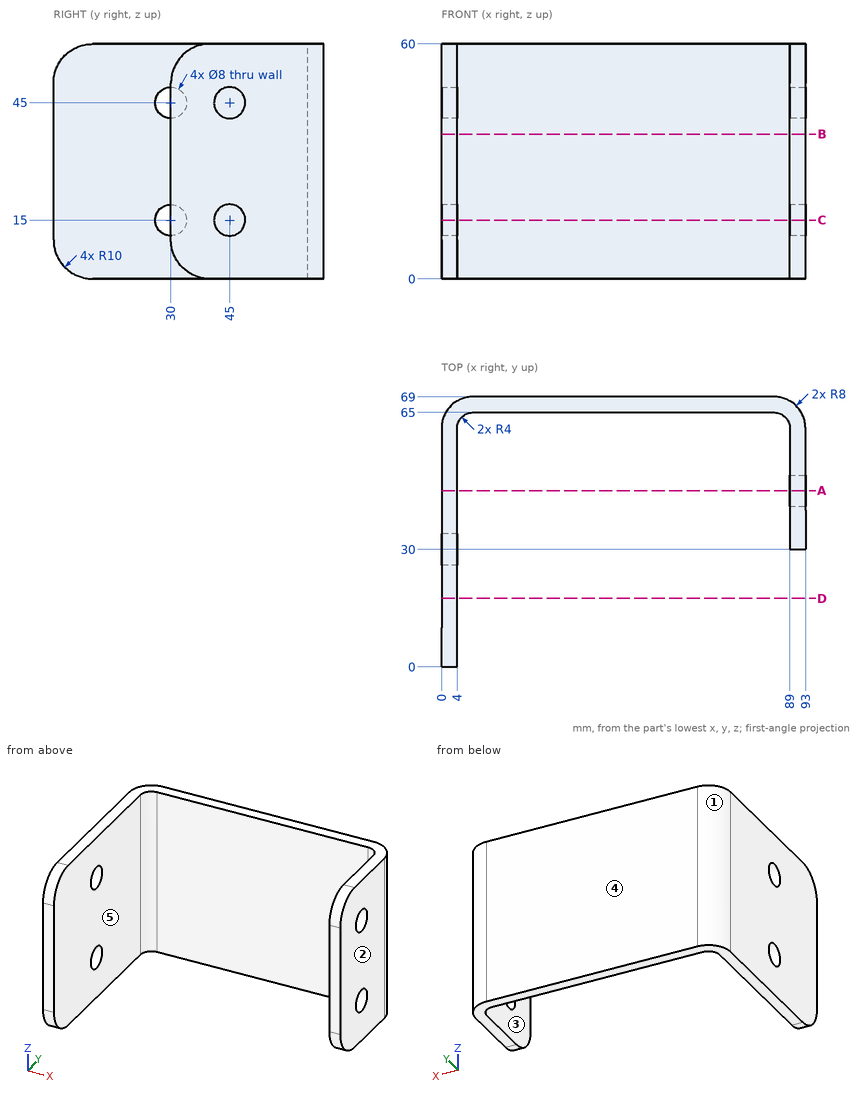
Geometry check sheet. Reference: drawing and pictorial views, mm from the part's lowest x, y, z. A direction names the side the tool comes from. Give positions to 0.01 mm unless a question says otherwise; leave off trailing zeros. Write each loop counter-clockwise with the first axis right and the second up, starting at its lowest first coordinate (ties: lowest second). Pieces come first, ordered by that corner, then holes.
Item 1: Cross-section at B-B (z = 37). Enter the section's corners in (x, y).
Item 2: Gauge pin test, flat ends, axial feed: pin 1 (6 mm diameter, centred on x = 40.5, z = 53.5, fed in from -Y); pin 2 (6.5 mm diameter, centred on y = 30, z = 45, fed in from -X); pin 3 (1 mm diameter, centred on y = 24.5, z = 40, fed in from +X). Record the tip position at first contact, or that the pin passes through.
Item 3: Access from +Z, -Z, +X, -X, +Y, -Y to the whole of each face (thin tool, end or side, straight path). Record for the marked faces 4 and 5.
Item 4: Cross-section at D-D (y = 17.5). Enter the section's corners in (x, z), and give its area (3 significant figures).
Item 5: Cross-section at C-C (z = 15). Enter the section's corners in (x, y).
Item 6: Draft check along X on the marked faces 1, 2 and 3. Enter one of: released by +X, released by -X, zero draft, split by the parting line, or undercut.
Item 7: Scan lines: L1, parallel to X at y = 45, z = 4.5; L2, parallel to X at y = 28.5, z = 29.5; L3, parallel to Y at x = 91, z = 45. Record each from-to range of solid material in increasing order.
Item 8: Cross-section at A-A (y = 45). Enter the section's corners in (x, z), and give its area (3 significant figures).
Report:
1. outline: (0, 0) - (4, 0) - (4, 61) arc R4 cw to (8, 65) - (85, 65) arc R4 cw to (89, 61) - (89, 30) - (93, 30) - (93, 61) arc R8 ccw to (85, 69) - (8, 69) arc R8 ccw to (0, 61) - close
2. pin 1: stops at y = 65
2. pin 2: stops at x = 89
2. pin 3: stops at x = 4
3. face 4: +Z, -Z, +X, -X, +Y
3. face 5: +Z, -Z, -Y
4. outline: (0, 0) - (4, 0) - (4, 60) - (0, 60) - close
4. area: 240 mm2
5. outline: (0, 0) - (4, 0) - (4, 26) - (0, 26) - close; (0, 34) - (4, 34) - (4, 61) arc R4 cw to (8, 65) - (85, 65) arc R4 cw to (89, 61) - (89, 49) - (93, 49) - (93, 61) arc R8 ccw to (85, 69) - (8, 69) arc R8 ccw to (0, 61) - close; (89, 30) - (93, 30) - (93, 41) - (89, 41) - close
6. face 1: released by -X
6. face 2: released by +X
6. face 3: undercut
7. L1: x = 0 to 4, 89 to 93
7. L2: x = 0 to 4
7. L3: y = 30 to 41, 49 to 66.29
8. outline: (0, 0) - (4, 0) - (4, 60) - (0, 60) - close; (89, 0) - (93, 0) - (93, 11) - (89, 11) - close; (89, 19) - (93, 19) - (93, 41) - (89, 41) - close; (89, 49) - (93, 49) - (93, 60) - (89, 60) - close
8. area: 416 mm2
